Model file for the job. Use its own axes, mm. A direction names the side the tool comes from. Round coordinates to 2 decimals unless told otherwise and drop trailing zeros. Order: outer loops, then holes, each group sorted by start corner. A loop starts at its lowest first (then second) coordinate and runs counter-clockwise, first axis right, second up. Notation, with made-up numbers: M -1.5,85.5 L 36.5,85.5 A14 cw 36.5,110.5 Z; hole C -38,46 d4. An arc over 180 degrees is marked long. Return JSON: item names as keys, results as strings. Group by question number.
Item 1: Probe line 1 along Z through (x, y) = (15.5, 31.5); line 2 along Y through (x, z) = (-15, 53.5); line 3 along Z through (x, y) = (-12, 1). List the from-to ranges inside material, lowest first.
Item 2: Slice it at A-A on y = 62.5. Write the cut outline in (x, z).
Item 3: Slice it at D-D on y = 50. Write the cut outline in (x, z), then the cut area to 3 significant figures.
Item 4: Slice it at C-C on x = 14. Write the cut outline in (y, z) (3 decimals), then the cut area to 3 significant figures.
Item 5: Slice it at B-B on x = 0. Write the cut outline in (y, z), then the cut area to 3 significant figures.
Item 6: Pin check, flat tips, straight feed: pin 1 Ø5 at (x, y) = (0, 38) entering from -Z; pin 2 Ø1.5 at (y, z) = (68.5, 1) entering from -X; pin 3 Ø6 at (x, z) = (-12.5, 31.565) entering from +Y; pin 4 Ø1.5 at (y, z) = (68.5, 60) entering from +X. Stop position of each tip, or through.
Item 7: Which spindle directions (+Z, -Z, +X, -X, +Y, -Y) get a long thin tool onto all of the face, cutting with end or side? Do faces 1 (the face through (0, 38, 59.13)), 2 (the face through (8, 70, 61)), 3 (the face through (2.998, 69, 61)). Say none if no direction does.
Item 8: Pull direction Z, two halves, no side cores. Call faces 4 (the face through (-16.198, 37.955, 1.972)), 5 (the face through (10.98, 2.54, 29.58)): pulls with the +Z half, pulls with the -Z half, needs draft (parallel to the pull), parting line crosses it, or undercut.
from build123d import *

# Parameters (mm, degrees)
ESTRUSIONE_ESTRUSIONE1_DEPTH = 4
SCHIZZO2_W                   = 40
SCHIZZO2_H                   = 5
ESTRUSIONE_ESTRUSIONE2_DEPTH = 55.13
ESTRUSIONE_ESTRUSIONE3_DEPTH = 4
SCHIZZO4_R                   = 2.5
TAGLIO_ESTRUSIONE1_DEPTH     = 93.792224351


with BuildPart() as part:
    # Schizzo1 → Estrusione-Estrusione1 (new body)
    with BuildSketch(Plane.XY):
        with BuildLine():
            Line((-20, 0), (20, 0))
            Line((20, 0), (20, 5))
            Line((20, 5), (12.5, 70))
            Line((12.5, 70), (2.997785692, 70))
            Line((2.997785692, 70), (2.997785692, 67))
            ThreePointArc((2.997785692, 67), (0, 64.002214308), (-2.997785692, 67))
            Line((-2.997785692, 67), (-2.997785692, 70))
            Line((-2.997785692, 70), (-12.5, 70))
            Line((-12.5, 70), (-20, 5))
            Line((-20, 5), (-20, 0))
        make_face()
    extrude(amount=ESTRUSIONE_ESTRUSIONE1_DEPTH)

    # Schizzo2 → Estrusione-Estrusione2 (add)
    with BuildSketch(Plane.XY.offset(4)):
        with Locations((0, 2.5)):
            Rectangle(SCHIZZO2_W, SCHIZZO2_H)
    extrude(amount=ESTRUSIONE_ESTRUSIONE2_DEPTH)

    # Schizzo3 → Estrusione-Estrusione3 (add)
    with BuildSketch(Plane.XY.offset(59.13)):
        with BuildLine():
            Line((20, 5), (12.5, 70))
            Line((12.5, 70), (2.997785692, 70))
            Line((2.997785692, 70), (2.997785692, 67))
            ThreePointArc((2.997785692, 67), (0, 64.002214308), (-2.997785692, 67))
            Line((-2.997785692, 67), (-2.997785692, 70))
            Line((-2.997785692, 70), (-12.5, 70))
            Line((-12.5, 70), (-20, 5))
            Line((-20, 5), (-20, 0))
            Line((-20, 0), (20, 0))
            Line((20, 0), (20, 5))
        make_face()
    extrude(amount=ESTRUSIONE_ESTRUSIONE3_DEPTH)

    # Schizzo4 → Taglio-Estrusione1 (cut, through all)
    with BuildSketch(Plane(origin=(0, 5, 0), x_dir=(1, 0, 0), z_dir=(0, 1, 0))):
        with Locations(Location((12.5, -31.565, 0), (0, 0, 270))):
            Circle(SCHIZZO4_R)
        with Locations(Location((-12.5, -31.565, 0), (0, 0, 270))):
            Circle(SCHIZZO4_R)
    extrude(amount=-TAGLIO_ESTRUSIONE1_DEPTH, mode=Mode.SUBTRACT)


solid = part.part
Output values:
{
 "1": {"line 1": "0 to 4, 59.13 to 63.13", "line 2": "0 to 5", "line 3": "0 to 29.12, 34.01 to 63.13"},
 "2": {"outline": "M -13.37,0 L 13.37,0 L 13.37,4 L -13.37,4 Z; M -13.37,59.13 L 13.37,59.13 L 13.37,63.13 L -13.37,63.13 Z"},
 "3": {"outline": "M -14.81,0 L 14.81,0 L 14.81,4 L -14.81,4 Z; M -14.81,59.13 L 14.81,59.13 L 14.81,63.13 L -14.81,63.13 Z", "area": "237 mm²"},
 "4": {"outline": "M 0,0 L 57,0 L 57,4 L 5,4 L 5,29.565 L 0,29.565 Z; M 0,33.565 L 5,33.565 L 5,59.13 L 57,59.13 L 57,63.13 L 0,63.13 Z", "area": "712 mm²"},
 "5": {"outline": "M 0,0 L 64,0 L 64,4 L 5,4 L 5,59.13 L 64,59.13 L 64,63.13 L 0,63.13 Z", "area": "788 mm²"},
 "6": {"pin 1": "z = 0", "pin 2": "x = -12.76", "pin 3": "y = 5", "pin 4": "x = 12.76"},
 "7": {"face 1": "+X, -X, +Y", "face 2": "+Z, -Z, +X, -X, +Y", "face 3": "+Z, -Z, +Y"},
 "8": {"face 4": "needs draft", "face 5": "undercut"}
}
